```python
from build123d import *

# Parameters (mm, degrees)
ESTRUSIONE_ESTRUSIONE3_DEPTH = 1.2
SCHIZZO3_R                   = 1.8
TAGLIO_ESTRUSIONE1_DEPTH     = 50
SCHIZZO4_R                   = 0.5
ESTRUSIONE_ESTRUSIONE4_DEPTH = 1


with BuildPart() as part:
    # Schizzo2 → Estrusione-Estrusione3 (new body, symmetric)
    with BuildSketch(Plane(origin=(0, 0, 0), x_dir=(1, 0, 0), z_dir=(0, 1, 0))):
        Polygon((3.175426481, 0), (1.58771324, 2.75), (-1.58771324, 2.75), (-3.175426481, 0), (-1.58771324, -2.75), (1.58771324, -2.75), align=None)
    extrude(amount=ESTRUSIONE_ESTRUSIONE3_DEPTH, both=True)

    # Schizzo3 → Taglio-Estrusione1 (cut, symmetric)
    with BuildSketch(Plane(origin=(0, 1.2, 0), x_dir=(1, 0, 0), z_dir=(0, 1, 0))):
        Circle(SCHIZZO3_R)
    extrude(amount=TAGLIO_ESTRUSIONE1_DEPTH, both=True, mode=Mode.SUBTRACT)

    # Schizzo4 → Estrusione-Estrusione4 (add)
    with BuildSketch(Plane(origin=(-2.38156986, 0, 1.375), x_dir=(0.5, 0, 0.866025404), z_dir=(-0.866025404, 0, 0.5))):
        Circle(SCHIZZO4_R)
    extrude(amount=ESTRUSIONE_ESTRUSIONE4_DEPTH)


solid = part.part
```
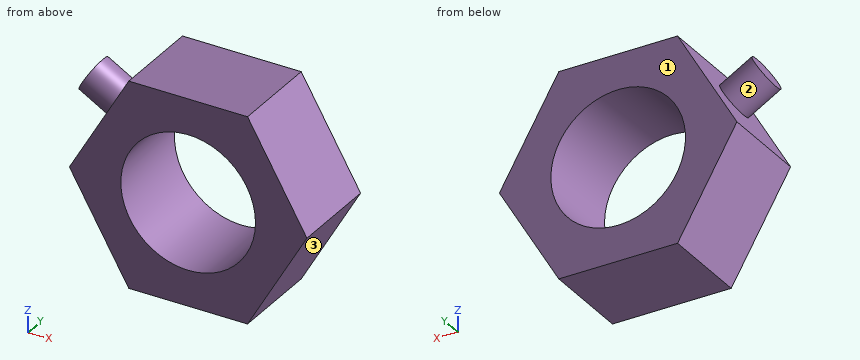
Input: part model. Units: mm. Frame: model coordinates. Face numbers are marked on the shaded views. Round coordinates to 2 decimals unless told otherwise and drop trailing zeros. Write each loop counter-clockwise with the first axis right and the second up, starting at its lowest first coordinate (ties: lowest second). Pieces come first, ordered by that corner, then holes. Notation, with made-up numbers: (83.5, 36) - (134.5, 36) arc R21 ccw to (134.5, 63) - close; hole circle Ø5 at (42.25, 20.25). An arc over 180 degrees is marked (long way). Write item = value, one per line.
(1) Section query D-D on x = -2. Output: boundary loops of the cut face in (y, z).
Geometry check:
outline = (-1.2, -2.04) - (1.2, -2.04) - (1.2, 2.04) - (-1.2, 2.04) - close
(2) Pull-direction query (X, two-part tool) for the marked faces 1, 2 and 3; classes: +X half, -X half, draft (parallel to the pull), parting line (faces both ways), or undercut.
Geometry check:
face_1 = draft
face_2 = undercut
face_3 = +X half
(3) Material intervals for probe 1 along Z at (x, y) = (0, -0.6); probe 2 along Z at (x, y) = (0.5, 0.8); probe 3 along X at (y, z) = (-0.7, -0.5), sorted ascending.
Geometry check:
probe_1 = -2.75 to -1.8, 1.8 to 2.75
probe_2 = -2.75 to -1.73, 1.73 to 2.75
probe_3 = -2.89 to -1.73, 1.73 to 2.89
(4) Section query C-C on z = 0.5. Output: boundary loops of the cut face in (x, y).
Geometry check:
outline = (-2.89, -1.2) - (-1.73, -1.2) - (-1.73, 1.2) - (-2.89, 1.2) - close; (1.73, -1.2) - (2.89, -1.2) - (2.89, 1.2) - (1.73, 1.2) - close
(5) Section query A-A on x = 0. Output: boundary loops of the cut face in (y, z).
Geometry check:
outline = (-1.2, -2.75) - (1.2, -2.75) - (1.2, -1.8) - (-1.2, -1.8) - close; (-1.2, 1.8) - (1.2, 1.8) - (1.2, 2.75) - (-1.2, 2.75) - close
(6) Section query B-B on y = -0.95. Output: boundary loops of the cut face in (x, z).
Geometry check:
outline = (-3.18, 0) - (-1.59, -2.75) - (1.59, -2.75) - (3.18, 0) - (1.59, 2.75) - (-1.59, 2.75) - close; hole circle Ø3.6 at (0, 0)
(7) Contact query for a flat-ended pin moving along its axis: pin 1 Ø3 at (x, z) = (0, 0) entering from -Y. Output: stop coordinate, or through.
Geometry check:
pin_1 = through
